Can you work these out from the drawing? Everything is in mm from the part's minimum corner. A direction names the side the tool comes from. Round coordinates to 2 decimals unless told otherwise and drop trailing zeros. Order: outer loops, then holes, each group sorted by start corner. A loop starts at its lowest first (then second) coordinate and runs counter-clockwise, first axis right, second up. Notation, with made-up numbers: M -19,-31 L 26,-31 A9 cw 26,-23 Z; hole C 11.25,-4 d3. An arc over 180 degrees is marked long. Use one line per item in the form item = value. Start each with the question number.
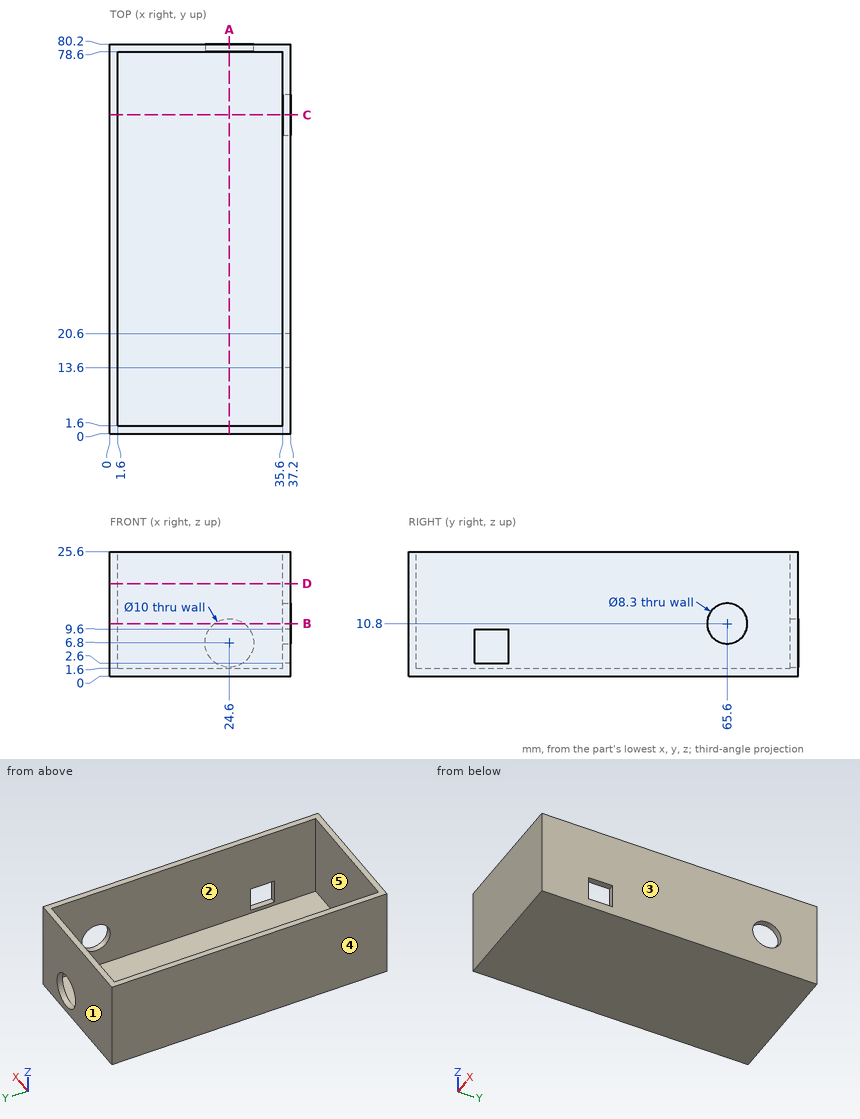
1) Will this pin go through, and if not, where does the flat tip stop? pin 1 Ø2 at (x, y) = (32.5, 30) entering from +Z.
2) If we mould it in two halves opening along X, with no side actions, what happens to the marked faces 1, 2 and 3? For each: +X half, -X half, draft (parallel to the pull), parting line (faces both ways), or undercut.
3) If we section it at A-A on x = 24.6: Write out the boundary of the cut face in (y, z).
4) On a 3-axis mill with a long thin cutter (end or side, diameter ignored), from which of +Z, -Z, +X, -X, +Y, -Y can I reach the whole of each face in a straight line? I mean the marked faces 4 and 5. Say none if no direction works.
5) If we section it at D-D on z = 19: Write out the boundary of the cut face in (x, y), then the cut area to 3 significant figures.
6) If we section it at B-B on z = 10.8: Write out the boundary of the cut face in (x, y).
7) If I drill on line 1 (X direction, y = 45, z = 16.75); line 2 (Y direction, x = 31, z = 14.75); line 3 (Z direction, x = 24.6, y = 79.35), over which ranges is the centre line in solid material (lowest first)?
8) If we section it at C-C on y = 65.6: Write out the boundary of the cut face in (x, z), then the cut area to 3 significant figures.
Completed:
q1.pin_1 = 1.6
q2.face_1 = draft
q2.face_2 = undercut
q2.face_3 = +X half
q3.outline = M 0,0 L 80.2,0 L 80.2,1.8 L 78.6,1.8 L 78.6,1.6 L 1.6,1.6 L 1.6,25.6 L 0,25.6 Z; M 78.6,11.8 L 80.2,11.8 L 80.2,25.6 L 78.6,25.6 Z
q4.face_4 = +Z, -Z, -X, +Y, -Y
q4.face_5 = +Z
q5.outline = M 0,0 L 37.2,0 L 37.2,80.2 L 0,80.2 Z; hole M 1.6,1.6 L 35.6,1.6 L 35.6,78.6 L 1.6,78.6 Z
q5.area = 365 mm²
q6.outline = M 0,0 L 37.2,0 L 37.2,61.45 L 35.6,61.45 L 35.6,1.6 L 1.6,1.6 L 1.6,78.6 L 21.6,78.6 L 21.6,80.2 L 0,80.2 Z; M 27.6,78.6 L 35.6,78.6 L 35.6,69.75 L 37.2,69.75 L 37.2,80.2 L 27.6,80.2 Z
q7.line_1 = 0 to 1.6, 35.6 to 37.2
q7.line_2 = 0 to 1.6, 78.6 to 80.2
q7.line_3 = 0 to 1.8, 11.8 to 25.6
q8.outline = M 0,0 L 37.2,0 L 37.2,6.65 L 35.6,6.65 L 35.6,1.6 L 1.6,1.6 L 1.6,25.6 L 0,25.6 Z; M 35.6,14.95 L 37.2,14.95 L 37.2,25.6 L 35.6,25.6 Z
q8.area = 123 mm²
